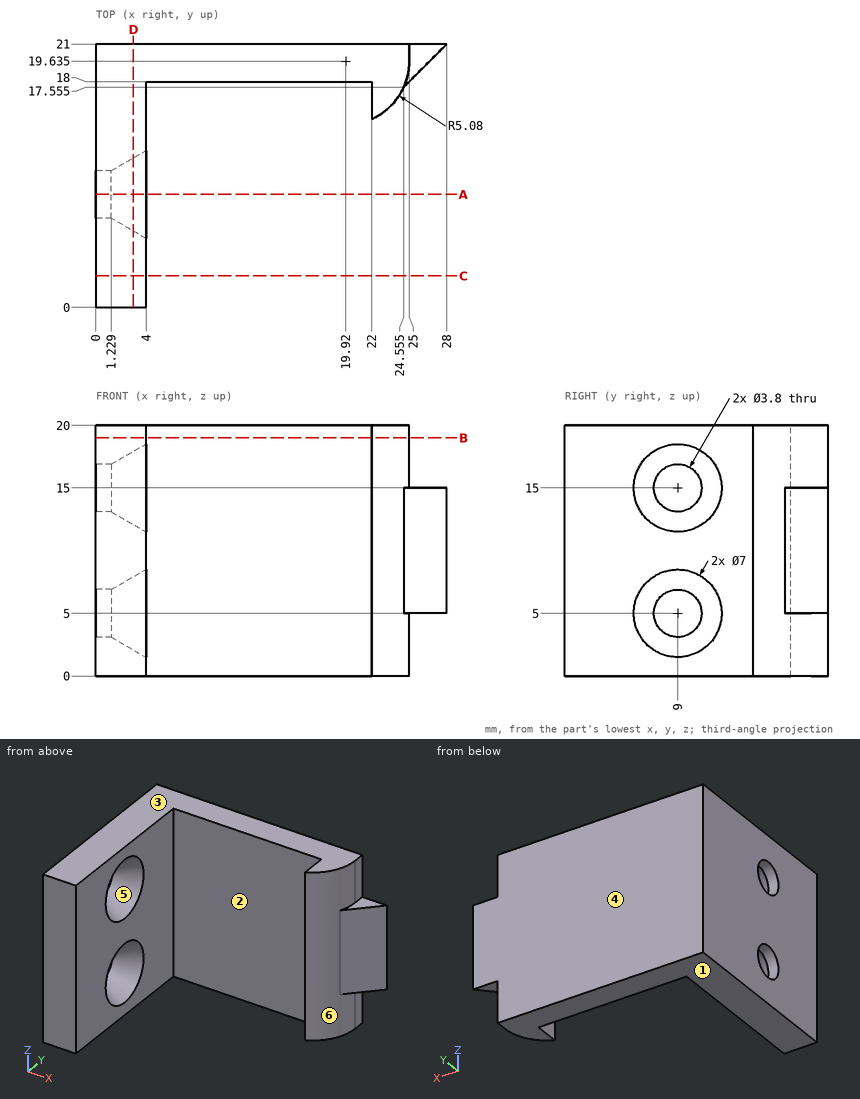
Geometry: see drawing. Coordinates: mm, zero at the bounding-box minimum. A direction names the side the tool comes from. Round coordinates to 2 decimals unless told otherwise and drop trailing zeros. Loops run counter-clockwise (first coordinate to the right, second up) from the corner with the lowest first, then second, coordinate; pieces in that order, holes last. Notation, with made-up numbers: M 45.5,16.5 L 99.5,16.5 A28 cw 99.5,35.5 Z; hole C 1,67 d5. An arc over 180 degrees is marked long. Use a Markdown table: item, result. Add a question column.
1. Section query C-C on y = 2.5. Return the cut outline in (x, z).
2. Line query: line 1 (Z direction, x = 0.45, y = 9); line 2 (Y direction, x = 0.8, z = 5); line 3 (X direction, y = 5.75, z = 2.5). Output: solid intervals per line, ascending.
3. Contact query for flat-ended pins moving along their axis: P1, Ø1.5, axis at x = 22, y = 12.5, coming from the +Z side; P2, Ø0.7, axis at y = 20, z = 18, coming from the +X side; P3, Ø3.5, axis at y = 16, z = 5.5, coming from the -X side; P4, Ø1.7, axis at x = 26, y = 19.5, coming from the -Z side. Output: stop coordinate, or through.
4. Section query B-B on z = 19. Return the cut outline in (x, y) (1 decimal), then the cut area to 3 significant figures.
5. Reachability of the marked faces 1 and 2 from +Z, -Z, +X, -X, +Y, -Y: full face, straight path, thin tool, end or side. Return the list, or none.
6. Section query D-D on x = 3. Return the cut outline in (y, z) (1 decimal), then the cut area to 3 significant figures.
7. Section query A-A on y = 9. Return the cut outline in (x, z).
8. Mould query, pull axis Y, two halves, no side actions, for the marked faces 3, 4, 5 and 6. Classes: pulls with the +Y half, pulls with the -Y half, needs draft (parallel to the pull), parting line crosses it, or undercut.
Reported:
| question | item | result |
|---|---|---|
| 1 | outline | M 0,0 L 4,0 L 4,20 L 0,20 Z |
| 2 | line 1 | z = 0 to 3.1, 6.9 to 13.1, 16.9 to 20 |
| 2 | line 2 | y = 0 to 7.1, 10.9 to 21 |
| 2 | line 3 | x = 0 to 4 |
| 3 | P1 | passes through |
| 3 | P2 | stops at x = 25 |
| 3 | P3 | stops at x = 0 |
| 3 | P4 | stops at z = 5 |
| 4 | outline | M 0,0 L 4,0 L 4,18 L 22,18 L 22,15 A5.1 ccw 25,19.6 L 25,21 L 0,21 Z |
| 4 | area | 152 mm² |
| 5 | face 1 | -Z, +X, -X, +Y, -Y |
| 5 | face 2 | +Z, -Z, -Y |
| 6 | outline | M 0,0 L 21,0 L 21,20 L 0,20 Z; hole C 9,5 d5.8; hole C 9,15 d5.8 |
| 6 | area | 366 mm² |
| 7 | outline | M 0,0 L 4,0 L 4,1.5 L 1.23,3.1 L 0,3.1 Z; M 0,6.9 L 1.23,6.9 L 4,8.5 L 4,11.5 L 1.23,13.1 L 0,13.1 Z; M 0,16.9 L 1.23,16.9 L 4,18.5 L 4,20 L 0,20 Z |
| 8 | face 3 | needs draft |
| 8 | face 4 | pulls with the +Y half |
| 8 | face 5 | undercut |
| 8 | face 6 | pulls with the -Y half |
